Part model, mm, in its own coordinate system. Face numbers are marked on the shaded views. A direction names the side the tool comes from. Give positions to 0.01 mm unless a question says otherwise; leave off trailing zeros. Write each loop counter-clockwise with the first axis right and the second up, starting at its lowest first coordinate (ties: lowest second). Pieces come first, ordered by that corner, then holes. Notation, with made-up numbers: M -35.5,-1.5 L -4.5,-1.5 A30 cw -4.5,37.5 Z; hole C 15.25,-4.5 d6. An arc over 180 degrees is marked long. Answer as CSV lines item,"result". Start each with the question number.
Item 1: 3-axis set-ups, long thin cutter, end or side, ignore diameter. For the marked faces 1, 2 and 3: which of +Z, -Z, +X, -X, +Y, -Y reach the whole face in a straight line?
Item 2: Wall check: L1, parallel to Y at x = 0, z = -1.7; L2, parallel to Y at x = 0, z = -6.25; L3, parallel to X at y = -0.5, z = -5.5. Give the ranges that are in metal, low to high. Write a range as from..to.
Item 3: Band-saw the part on D-D, the plane y = 2. List the corners of the cut face in (x, z) (3 decimals), then the cut area to 3 significant figures.
Item 4: Pin check, flat tips, straight feed: pin 1 (3 mm diameter, centred on y = -2.5, z = 3.5, fed in from +X); pin 2 (1.1 mm diameter, centred on x = -0.5, y = -1, fed in from +Z); pin 3 (3 mm diameter, centred on x = 0, y = 0, fed in from -Z); pin 4 (1.6 mm diameter, centred on x = 0, y = 0, fed in from -Z). Stop position of each tip, or through.
Item 5: Band-saw the part on A-A, the plane x = 0. List the corners of the cut face in (y, z) (3 decimals).
Item 6: Band-saw the part on C-C, the plane z = 6.5. List the corners of the cut face in (x, y), then the cut area to 3 significant figures.
from build123d import *

# Parameters (mm, degrees)
SKETCH1_R                       = 3.96875
BOSS_EXTRUDE1_DEPTH             = 9.525
F_6_32_TAPPED_HOLE1_D           = 2.7051
F_6_32_TAPPED_HOLE1_DEPTH       = 9.398
F_6_32_TAPPED_HOLE1_CBORE_D     = 3.5052
F_6_32_TAPPED_HOLE1_CBORE_DEPTH = 7.112
F_6_32_TAPPED_HOLE1_TIP         = 0.81269403
F_6_32_TAPPED_HOLE2_D           = 2.7051
F_6_32_TAPPED_HOLE2_DEPTH       = 9.398
F_6_32_TAPPED_HOLE2_CBORE_D     = 3.5052
F_6_32_TAPPED_HOLE2_CBORE_DEPTH = 7.112
F_6_32_TAPPED_HOLE2_TIP         = 0.81269403


with BuildPart() as part:
    # Sketch1 → Boss-Extrude1 (new, symmetric)
    with BuildSketch(Plane.XY):
        with Locations(Location((0, 0, 0), (0, 0, 180))):
            Circle(SKETCH1_R)
    extrude(amount=BOSS_EXTRUDE1_DEPTH, both=True)

    # #6-32 Tapped Hole1
    with Locations(Plane(origin=(0, 0, -9.525), x_dir=(-1, 0, 0), z_dir=(0, 0, -1))):
        with Locations((0, 0)):
            CounterBoreHole(F_6_32_TAPPED_HOLE1_D / 2, F_6_32_TAPPED_HOLE1_CBORE_D / 2, F_6_32_TAPPED_HOLE1_CBORE_DEPTH, depth=F_6_32_TAPPED_HOLE1_DEPTH)
            with Locations((0, 0, -(F_6_32_TAPPED_HOLE1_DEPTH + F_6_32_TAPPED_HOLE1_TIP / 2))):  # 118° drill point
                Cone(0, F_6_32_TAPPED_HOLE1_D / 2, F_6_32_TAPPED_HOLE1_TIP, mode=Mode.SUBTRACT)

    # #6-32 Tapped Hole2
    with Locations(Plane.XY.offset(9.525)):
        with Locations((0, 0)):
            CounterBoreHole(F_6_32_TAPPED_HOLE2_D / 2, F_6_32_TAPPED_HOLE2_CBORE_D / 2, F_6_32_TAPPED_HOLE2_CBORE_DEPTH, depth=F_6_32_TAPPED_HOLE2_DEPTH)
            with Locations((0, 0, -(F_6_32_TAPPED_HOLE2_DEPTH + F_6_32_TAPPED_HOLE2_TIP / 2))):  # 118° drill point
                Cone(0, F_6_32_TAPPED_HOLE2_D / 2, F_6_32_TAPPED_HOLE2_TIP, mode=Mode.SUBTRACT)


solid = part.part
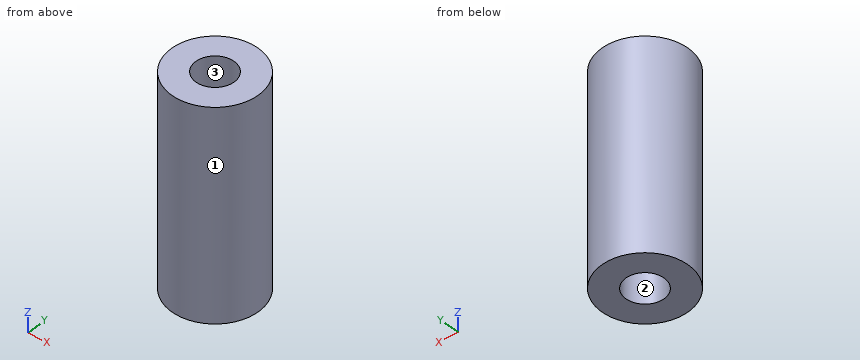
Output:
1,face 1,"+Z, -Z"
1,face 2,"-Z"
1,face 3,"+Z"
2,L1,"-3.97..-1.35, 1.35..3.97"
2,L2,"-3.97..-1.75, 1.75..3.97"
2,L3,"-3.94..-1.68, 1.68..3.94"
3,outline,"M -3.428,-9.525 L 3.428,-9.525 L 3.428,9.525 L -3.428,9.525 Z"
3,area,"131 mm²"
4,pin 1,"x = 3.84"
4,pin 2,"z = 2.41"
4,pin 3,"z = -2.41"
4,pin 4,"through"
5,outline,"M -3.969,-9.525 L -1.753,-9.525 L -1.753,-2.413 L -1.353,-2.413 L -1.353,-0.127 L -1.141,0 L -1.353,0.127 L -1.353,2.413 L -1.753,2.413 L -1.753,9.525 L -3.969,9.525 Z; M 1.141,0 L 1.353,-0.127 L 1.353,-2.413 L 1.753,-2.413 L 1.753,-9.525 L 3.969,-9.525 L 3.969,9.525 L 1.753,9.525 L 1.753,2.413 L 1.353,2.413 L 1.353,0.127 Z"
6,outline,"C 0,0 d7.94; hole C 0,0 d3.51"
6,area,"39.8 mm²"
